```python
from build123d import *

# Parameters (mm, degrees)
SKETCH1_W           = 236.22
SKETCH1_H           = 18.288
SKETCH1_R           = 9.652
BOSS_EXTRUDE1_DEPTH = 5
FILLET1_R           = 10
SKETCH2_W           = 216.043861244
SKETCH2_H           = 2.794
BOSS_EXTRUDE2_DEPTH = 7.62
SKETCH3_R           = 0.75
CUT_EXTRUDE1_DEPTH  = 5


with BuildPart() as part:
    # Sketch1 → Boss-Extrude1 (new body)
    with BuildSketch(Plane.XY):
        with Locations((118.11, 9.144)):
            Rectangle(SKETCH1_W, SKETCH1_H)
        with BuildLine():
            ThreePointArc((174.18, 5.144), (178.18, 9.144), (174.18, 13.144))
            Line((174.18, 13.144), (9.08, 13.144))
            ThreePointArc((9.08, 13.144), (5.08, 9.144), (9.08, 5.144))
            Line((9.08, 5.144), (174.18, 5.144))
        make_face(mode=Mode.SUBTRACT)
        Polygon((236.22, 18.288), (236.22, 0), (313.22, 0), (313.22, 50), (236.22, 50), align=None)
        with Locations((291.63, 28.638)):
            Circle(SKETCH1_R, mode=Mode.SUBTRACT)
    extrude(amount=BOSS_EXTRUDE1_DEPTH)

    # Fillet1
    fillet1_edges = [part.edges().sort_by_distance(p)[0] for p in [
        (236.22, 18.288, 2.5),
        (236.22, 50, 2.5),
        (313.22, 50, 2.5),
        (313.22, 0, 2.5),
    ]]
    fillet(fillet1_edges, radius=FILLET1_R)

    # Sketch2 → Boss-Extrude2 (add)
    with BuildSketch(Plane.XY.offset(5)):
        with Locations((108.021930622, 16.891)):
            Rectangle(SKETCH2_W, SKETCH2_H)
        with Locations((108.021930622, 1.397)):
            Rectangle(SKETCH2_W, SKETCH2_H)
    extrude(amount=BOSS_EXTRUDE2_DEPTH)

    # Sketch3 → Cut-Extrude1 (cut)
    with BuildSketch(Plane.XY.offset(12.62)):
        with Locations((2.5, 16.891)):
            Circle(SKETCH3_R)
        with Locations((2.5, 1.397)):
            Circle(SKETCH3_R)
        with Locations((107.6321922, 16.891)):
            Circle(SKETCH3_R)
        with Locations((107.6321922, 1.397)):
            Circle(SKETCH3_R)
        with Locations((213.543861244, 16.891)):
            Circle(SKETCH3_R)
        with Locations((213.543861244, 1.397)):
            Circle(SKETCH3_R)
    extrude(amount=-CUT_EXTRUDE1_DEPTH, mode=Mode.SUBTRACT)


solid = part.part
```
The model under review builds one solid part; all positions refer to its coordinate system, in mm. A direction names the side the tool comes from. Round coordinates to 2 decimals unless told otherwise and drop trailing zeros. Loops run counter-clockwise (first coordinate to the right, second up) from the corner with the lowest first, then second, coordinate; pieces in that order, holes last. Notation, with made-up numbers: (39, 39) -> (76, 39) arc R25 ccw to (76, 51) -> close; hole circle Ø8 at (-20, 45.25). An arc over 180 degrees is marked (long way). Answer as a JSON object with one key per item and string values. Group by question number.
1) For pin 1 Ø0.9 at (x, y) = (213.54, 1.4) entering from +Z; pin 2 Ø2.5 at (y, z) = (33, 2) entering from -X; pin 3 Ø1.5 at (x, z) = (108, 9.5) entering from +Y, all flat-tipped, find the tip position at first contact; note any pin that passes through.
2) For line 1 (Y direction, x = 2.5, z = 11.15); line 2 (X direction, y = 9.5, z = 3); line 3 (Y direction, x = 82.5, z = 4), list the stretches that pass through material, from the lowest coordinate up. Write a range as [from, to].
3) We need section A-A on z = 10.25. Write out the cut boundary in (x, y), then the cut area to 3 significant figures.
4) Mouldability with a two-part tool opening along Y and no side actions: class faces 6 (the face through (189, 14, 0)), 7 (the face through (300.836, 31.537, 2.465)), 8 (the face through (310.37, 46.99, 2.54)) as released by +Y, released by -Y, zero draft, split by the parting line, or undercut.
5) We need section D-D on y = 46.5. Write out the cut boundary in (x, z).
6) For faces 1 (the face through (5.08, 9.23, 2.46)), 2 (the face through (0, 9, 3)), 3 (the face through (107, 2.794, 9)), 4 (the face through (116, 0, 6)), 5 (the face through (236.22, 34, 2)), list the 3-axis set-ups (+Z, -Z, +X, -X, +Y, -Y) from which the entire face can be reached by the end or side of a thin tool; tool diameter is ignored.
7) We need section C-C on y = 35. Write out the cut boundary in (x, z), then the cut area to 3 significant figures.
8) We need section B-B on x = 291.63. Write out the cut boundary in (y, z).
Result set:
{
 "1": {"pin 1": "z = 7.62", "pin 2": "x = 236.22", "pin 3": "y = 18.29"},
 "2": {"line 1": "[0, 0.65], [2.15, 2.79], [15.49, 16.14], [17.64, 18.29]", "line 2": "[0, 5.1], [178.16, 313.21]", "line 3": "[0, 5.14], [13.14, 18.29]"},
 "3": {"outline": "(0, 0) -> (216.04, 0) -> (216.04, 2.79) -> (0, 2.79) -> close; (0, 15.49) -> (216.04, 15.49) -> (216.04, 18.29) -> (0, 18.29) -> close; hole circle Ø1.5 at (2.5, 1.4); hole circle Ø1.5 at (2.5, 16.89); hole circle Ø1.5 at (107.63, 1.4); hole circle Ø1.5 at (107.63, 16.89); hole circle Ø1.5 at (213.54, 1.4); hole circle Ø1.5 at (213.54, 16.89)", "area": "1,200 mm²"},
 "4": {"face 6": "zero draft", "face 7": "undercut", "face 8": "released by +Y"},
 "5": {"outline": "(238.62, 0) -> (310.82, 0) -> (310.82, 5) -> (238.62, 5) -> close"},
 "6": {"face 1": "+Z, -Z", "face 2": "+Z, -Z, -X, +Y, -Y", "face 3": "+Z, +X, -X", "face 4": "+Z, -Z, +X, -X, -Y", "face 5": "+Z, -Z, -X, +Y"},
 "7": {"outline": "(236.22, 0) -> (284.37, 0) -> (284.37, 5) -> (236.22, 5) -> close; (298.89, 0) -> (313.22, 0) -> (313.22, 5) -> (298.89, 5) -> close", "area": "312 mm²"},
 "8": {"outline": "(0, 0) -> (18.99, 0) -> (18.99, 5) -> (0, 5) -> close; (38.29, 0) -> (50, 0) -> (50, 5) -> (38.29, 5) -> close"}
}
